from build123d import *

# Parameters (mm, degrees)
ESBO_O1_W                = 35
ESBO_O1_H                = 25.1
RESSALTO_EXTRUS_O1_DEPTH = 2
ESBO_O2_R                = 1.5
CORTE_EXTRUS_O1_DEPTH    = 2
ESBO_O3_W                = 2.002857319
ESBO_O3_H                = 25.1
RESSALTO_EXTRUS_O2_DEPTH = 2
CORTE_EXTRUS_O2_DEPTH    = 2
ESBO_O5_W                = 4
ESBO_O5_H                = 25.1
RESSALTO_EXTRUS_O3_DEPTH = 2
ESBO_O6_W                = 41.002857319
ESBO_O6_H                = 25.1
RESSALTO_EXTRUS_O4_DEPTH = 10
ESBO_O7_W                = 17.37169178
ESBO_O7_H                = 25.1
RESSALTO_EXTRUS_O5_DEPTH = 2
ESBO_O8_R                = 1.5
CORTE_EXTRUS_O3_DEPTH    = 20
RESSALTO_EXTRUS_O6_START = -10
RESSALTO_EXTRUS_O6_DEPTH = 10
ESBO_O10_W               = 2
ESBO_O10_H               = 2
RESSALTO_EXTRUS_O7_DEPTH = 10
ESBO_O11_R               = 1.5
CORTE_EXTRUS_O4_DEPTH    = 15
ESBO_O12_W               = 41.002857319
ESBO_O12_H               = 1
RESSALTO_EXTRUS_O8_DEPTH = 12
CORTE_EXTRUS_O5_DEPTH    = 10
ESBO_O14_W               = 8
ESBO_O14_H               = 23.06
CORTE_EXTRUS_O6_DEPTH    = 10


with BuildPart() as part:
    # Esboço1 → Ressalto-extrusão1 (new body)
    with BuildSketch(Plane.XY):
        with Locations((17.5, 12.55)):
            Rectangle(ESBO_O1_W, ESBO_O1_H)
    extrude(amount=RESSALTO_EXTRUS_O1_DEPTH)

    # Esboço2 → Corte-extrusão1 (cut)
    with BuildSketch(Plane.XY.offset(2)):
        with Locations((2.13, 22.97)):
            Circle(ESBO_O2_R)
        with Locations(Location((2.13, 2.13, 0), (0, 0, 180))):
            Circle(ESBO_O2_R)
    extrude(amount=-CORTE_EXTRUS_O1_DEPTH, mode=Mode.SUBTRACT)

    # Esboço3 → Ressalto-extrusão2 (add)
    with BuildSketch(Plane.XY.offset(2)):
        with Locations((-1.00142866, 12.55)):
            Rectangle(ESBO_O3_W, ESBO_O3_H)
    extrude(amount=-RESSALTO_EXTRUS_O2_DEPTH)

    # Esboço4 → Corte-extrusão2 (cut)
    with BuildSketch(Plane.XY.offset(2)):
        Polygon((1.597142681, 12.55), (1.597142681, 19.05), (14.597142681, 19.05), (14.597142681, 6.05), (1.597142681, 6.05), align=None)
    extrude(amount=-CORTE_EXTRUS_O2_DEPTH, mode=Mode.SUBTRACT)

    # Esboço5 → Ressalto-extrusão3 (add)
    with BuildSketch(Plane.XY.offset(2)):
        with Locations((37, 12.55)):
            Rectangle(ESBO_O5_W, ESBO_O5_H)
    extrude(amount=-RESSALTO_EXTRUS_O3_DEPTH)

    # Esboço6 → Ressalto-extrusão4 (add)
    with BuildSketch(Plane(origin=(0, 0, 0), x_dir=(-1, 0, 0), z_dir=(0, 0, -1))):
        with Locations((-18.49857134, 12.55)):
            Rectangle(ESBO_O6_W, ESBO_O6_H)
        with BuildLine():
            Line((-32.997142681, 22.1), (-4, 22.1))
            ThreePointArc((-4, 22.1), (-2, 20.1), (0, 22.1))
            Line((0, 22.1), (0, 3))
            ThreePointArc((0, 3), (-2, 5), (-4, 3))
            Line((-4, 3), (-32.997142681, 3))
            ThreePointArc((-32.997142681, 3), (-34.997142681, 5), (-36.997142681, 3))
            Line((-36.997142681, 3), (-36.997142681, 22.1))
            ThreePointArc((-36.997142681, 22.1), (-34.997142681, 20.1), (-32.997142681, 22.1))
        make_face(mode=Mode.SUBTRACT)
    extrude(amount=RESSALTO_EXTRUS_O4_DEPTH)

    # Esboço7 → Ressalto-extrusão5 (add)
    with BuildSketch(Plane.XY.offset(2)):
        with Locations((6.682988571, 12.55)):
            Rectangle(ESBO_O7_W, ESBO_O7_H)
    extrude(amount=-RESSALTO_EXTRUS_O5_DEPTH)

    # Esboço8 → Corte-extrusão3 (cut)
    with BuildSketch(Plane(origin=(0, 0, -10), x_dir=(-1, 0, 0), z_dir=(0, 0, -1))):
        with Locations((-2, 22.585)):
            Circle(ESBO_O8_R)
        with Locations((-2, 2.515)):
            Circle(ESBO_O8_R)
    extrude(amount=-CORTE_EXTRUS_O3_DEPTH, mode=Mode.SUBTRACT)

    # Esboço9 → Ressalto-extrusão6 (add)
    with BuildSketch(Plane(origin=(0, 0, -10), x_dir=(-1, 0, 0), z_dir=(0, 0, -1)).offset(RESSALTO_EXTRUS_O6_START)):
        with BuildLine():
            Line((-2, 20.1), (0, 20.1))
            Line((0, 20.1), (0, 22.1))
            ThreePointArc((0, 22.1), (-0.585786438, 20.685786438), (-2, 20.1))
        make_face()
        with BuildLine():
            Line((0, 5), (0, 3))
            ThreePointArc((0, 3), (-0.585786438, 4.414213562), (-2, 5))
            Line((-2, 5), (0, 5))
        make_face()
    extrude(amount=RESSALTO_EXTRUS_O6_DEPTH)

    # Esboço10 → Ressalto-extrusão7 (add)
    with BuildSketch(Plane(origin=(0, 0, -10), x_dir=(-1, 0, 0), z_dir=(0, 0, -1))):
        Polygon((-34.997142681, 20.1), (-36.997142681, 20.1), (-36.997142681, 22.1), align=None)
        with Locations((-35.997142681, 4)):
            Rectangle(ESBO_O10_W, ESBO_O10_H)
    extrude(amount=-RESSALTO_EXTRUS_O7_DEPTH)

    # Esboço11 → Corte-extrusão4 (cut)
    with BuildSketch(Plane(origin=(0, 0, -10), x_dir=(-1, 0, 0), z_dir=(0, 0, -1))):
        with Locations((-34.997142681, 22.585)):
            Circle(ESBO_O11_R)
        with Locations((-34.997142681, 2.515)):
            Circle(ESBO_O11_R)
    extrude(amount=-CORTE_EXTRUS_O4_DEPTH, mode=Mode.SUBTRACT)

    # Esboço12 → Ressalto-extrusão8 (add)
    with BuildSketch(Plane(origin=(0, 0, -10), x_dir=(-1, 0, 0), z_dir=(0, 0, -1))):
        with Locations((-18.49857134, 25.6)):
            Rectangle(ESBO_O12_W, ESBO_O12_H)
        with Locations((-18.49857134, -0.5)):
            Rectangle(ESBO_O12_W, ESBO_O12_H)
    extrude(amount=-RESSALTO_EXTRUS_O8_DEPTH)

    # Esboço13 → Corte-extrusão5 (cut)
    with BuildSketch(Plane(origin=(0, 0, -10), x_dir=(-1, 0, 0), z_dir=(0, 0, -1))):
        Polygon((-2, 24.085), (0, 24.085), (0, 1.015), (-2, 1.015), (-36.997142681, 1.015), (-36.997142681, 24.085), align=None)
    extrude(amount=-CORTE_EXTRUS_O5_DEPTH, mode=Mode.SUBTRACT)

    # Esboço14 → Corte-extrusão6 (cut)
    with BuildSketch(Plane(origin=(39, 0, 0), x_dir=(0, 0, -1), z_dir=(1, 0, 0))):
        with Locations((4, 12.55)):
            Rectangle(ESBO_O14_W, ESBO_O14_H)
    extrude(amount=-CORTE_EXTRUS_O6_DEPTH, mode=Mode.SUBTRACT)


solid = part.part
Here's how the part is built. I have some questions about the finished solid (model axes, mm). A direction names the side the tool comes from. Round coordinates to 2 decimals unless told otherwise and drop trailing zeros. Order: outer loops, then holes, each group sorted by start corner. A loop starts at its lowest first (then second) coordinate and runs counter-clockwise, first axis right, second up. Notation, with made-up numbers: M 54.25,66.5 L 90.25,66.5 A31 cw 90.25,94.5 Z; hole C -29.5,-33.75 d3. An arc over 180 degrees is marked long. Return JSON: item names as keys, results as strings. Group by question number.
1. On a 3-axis mill with a long thin cutter (end or side, diameter ignored), from which of +Z, -Z, +X, -X, +Y, -Y can I reach the whole of each face in a straight line? I mean faces 4 (the face through (18, 24.085, -5)), 5 (the face through (38, 1.02, -4)), 6 (the face through (39, 12, -9)). Say none if no direction works.
2. If we section it at C-C on x = 7: List the corners of the cut face in (y, z) for me (3 decimals).
3. If we mould it in two halves opening along Y, with no side actions, what happens to faces 1 (the face through (19, 1.015, -5)), 2 (the face through (20.1, 0.6, -10)), 3 (the face through (19, -1, -4))? For each: pulls with the +Y half, pulls with the -Y half, needs draft (parallel to the pull), parting line crosses it, or undercut.
4. If we section it at B-B on z = -0.5: List the corners of the cut face in (x, y) for me (3 decimals).
5. If we section it at A-A on y = 8: List the corners of the cut face in (x, z) for me, then the cut area to 3 significant figures.
6. I'm going to push flat-ended pins straight in: pin 1 Ø4 at (y, z) = (4.5, -4) entering from +X; pin 2 Ø4 at (x, y) = (20, 18.5) entering from -Z. Where does each tip first touch, or does it pass through?
7. Please list where these lines run through material, in increasing order: probe 1 along Y at (x, z) = (18, -9.25) (3 decimals); probe 2 along X at (y, z) = (16, -9); probe 3 along Y at (x, z) = (2, 1.3) (3 decimals).
Reply:
{
 "1": {"face 4": "-Z", "face 5": "+X", "face 6": "+Z, -Z, +X, +Y, -Y"},
 "2": {"outline": "M -1,-10 L 1.015,-10 L 1.015,0 L 24.085,0 L 24.085,-10 L 26.1,-10 L 26.1,2 L -1,2 Z"},
 "3": {"face 1": "undercut", "face 2": "needs draft", "face 3": "pulls with the -Y half"},
 "4": {"outline": "M -2.003,-1 L 39,-1 L 39,1.02 L 36.997,1.02 L 36.997,1.015 L 0,1.015 L 0,24.085 L 36.997,24.085 L 36.997,24.08 L 39,24.08 L 39,26.1 L -2.003,26.1 Z"},
 "5": {"outline": "M -2,-10 L 0,-10 L 0,0 L 39,0 L 39,2 L -2,2 Z; M 37,-10 L 39,-10 L 39,-8 L 37,-8 Z", "area": "106 mm^2"},
 "6": {"pin 1": "x = 0", "pin 2": "z = 0"},
 "7": {"probe 1": "-1 to 1.015, 24.085 to 26.1", "probe 2": "-2 to 0, 37 to 39", "probe 3": "-1 to 1.015, 4.015 to 21.085, 24.085 to 26.1"}
}
